from build123d import *

# Parameters (mm, degrees)
SKETCH1_W           = 1050
SKETCH1_H           = 409.5
BOSS_EXTRUDE1_DEPTH = 1
SKETCH2_W           = 150
SKETCH2_H           = 50
CUT_EXTRUDE1_DEPTH  = 1
FILLET1_R           = 10


with BuildPart() as part:
    # Sketch1 → Boss-Extrude1 (new body)
    with BuildSketch(Plane(origin=(0, 0, 0), x_dir=(1, 0, 0), z_dir=(0, 1, 0))):
        with Locations((-18.909884175, 328.455718826)):
            Rectangle(SKETCH1_W, SKETCH1_H)
    extrude(amount=BOSS_EXTRUDE1_DEPTH)

    # Sketch2 → Cut-Extrude1 (cut)
    with BuildSketch(Plane(origin=(0, 1, 0), x_dir=(1, 0, 0), z_dir=(0, 1, 0))):
        with Locations((-18.909884175, 148.705718826)):
            Rectangle(SKETCH2_W, SKETCH2_H)
    extrude(amount=-CUT_EXTRUDE1_DEPTH, mode=Mode.SUBTRACT)

    # Fillet1
    fillet1_edges = [part.edges().sort_by_distance(p)[0] for p in [
        (-93.909884175, 0.5, -173.705718826),
        (56.090115825, 0.5, -173.705718826),
    ]]
    fillet(fillet1_edges, radius=FILLET1_R)


solid = part.part
Read the model definition and answer for the solid it produces. Units are mm, in the model's axes. Coordinates: 2 decimals unless noted, no trailing zeros. Order: outer loops, then holes, each group sorted by start corner. A loop starts at its lowest first (then second) coordinate and runs counter-clockwise, first axis right, second up. Notation, with made-up numbers: M -21.75,78 L -11.75,78 A27 ccw -11.75,117 Z; hole C -19.5,31 d3. An arc over 180 degrees is marked long. Put each result on its own line as item: value. Start each with the question number.
Item 1: Section B-B, the plane y = 0.7 is taken. Determine the outline of the cut face in (x, z).
Item 2: Section A-A, the plane z = -150.5 is taken. Determine the outline of the cut face in (x, y).
Item 3: Section C-C, the plane x = -47 is taken. Determine the outline of the cut face in (y, z), plus the area to 4 significant figures.
Item 4: Consider probe 1 along Z at (x, y) = (-70, 0.95); probe 2 along X at (y, z) = (0.55, -169); probe 3 along Z at (x, y) = (-91.5, 0.8). Determine where each line is inside the solid, lowest interval first. Write a range as [from, to].
Computed:
1. outline: M -543.91,-533.21 L 506.09,-533.21 L 506.09,-123.71 L 56.09,-123.71 L 56.09,-163.71 A10 cw 46.09,-173.71 L -83.91,-173.71 A10 cw -93.91,-163.71 L -93.91,-123.71 L -543.91,-123.71 Z
2. outline: M -543.91,0 L -93.91,0 L -93.91,1 L -543.91,1 Z; M 56.09,0 L 506.09,0 L 506.09,1 L 56.09,1 Z
3. outline: M 0,-533.21 L 1,-533.21 L 1,-173.71 L 0,-173.71 Z
3. area: 359.5 mm2
4. probe 1: z = [-533.21, -173.71]
4. probe 2: x = [-543.91, -92.39], [54.57, 506.09]
4. probe 3: z = [-533.21, -170.22]
